```python
from build123d import *

# Parameters (mm, degrees)
BASPROSKE_W          = 4
BASPROSKE_H          = 12.375
TOOTHCUT_DEPTH       = 18.952193459
TEETHCUTS_COUNT      = 20
M2_CLEARANCE_HOLE1_D = 2.2
SKETCH3_R            = 2.5
CUT_EXTRUDE1_DEPTH   = 1


with BuildPart() as part:
    # BasProSke → Base-Revolve (revolve)
    with BuildSketch(Plane(origin=(0, 0, 0), x_dir=(1, 0, 0), z_dir=(0, 1, 0)), mode=Mode.PRIVATE) as base_revolve_sk:
        with Locations((2, 6.1875)):
            Rectangle(BASPROSKE_W, BASPROSKE_H)
    revolve(base_revolve_sk.sketch.rotate(Axis((-10, 0, 0), (1, 0, 0)), 180), axis=Axis((-10, 0, 0), (1, 0, 0)))

    # TooCutSke → ToothCut (cut, through all)
    with BuildSketch(Plane(origin=(0, 0, 0), x_dir=(0, 0, -1), z_dir=(1, 0, 0))):
        with BuildLine():
            ThreePointArc((0.561279811, 9.826733564), (0, 9.84275), (-0.561279811, 9.826733564))
            ThreePointArc((-0.561279811, 9.826733564), (-0.925277854, 11.14210546), (-1.666860651, 12.287859689))
            ThreePointArc((-1.666860651, 12.287859689), (0, 12.4004), (1.666860651, 12.287859689))
            ThreePointArc((1.666860651, 12.287859689), (0.925277854, 11.14210546), (0.561279811, 9.826733564))
        make_face()
    toothcut = extrude(amount=TOOTHCUT_DEPTH, mode=Mode.SUBTRACT)

    # TeethCuts: ToothCut ×20 about axis
    teethcuts_axis = Axis((0, 0, 0), (1, 0, 0))
    for i in range(1, TEETHCUTS_COUNT):
        add(toothcut.rotate(teethcuts_axis, i * 360 / TEETHCUTS_COUNT), mode=Mode.SUBTRACT)

    # M2 Clearance Hole1 (through all)
    with Locations(Plane(origin=(4, 0, 0), x_dir=(0, 0, -1), z_dir=(1, 0, 0))):
        with Locations((0, 0)):
            Hole(M2_CLEARANCE_HOLE1_D / 2)

    # Sketch3 → Cut-Extrude1 (cut)
    with BuildSketch(Plane(origin=(4, 0, 0), x_dir=(0, 0, -1), z_dir=(1, 0, 0))):
        Circle(SKETCH3_R)
    extrude(amount=-CUT_EXTRUDE1_DEPTH, mode=Mode.SUBTRACT)


solid = part.part
```
Model file for the job. Use its own axes, mm. A direction names the side the tool comes from. Round coordinates to 2 decimals unless told otherwise and drop trailing zeros. Write each loop counter-clockwise with the first axis right and the second up, starting at its lowest first coordinate (ties: lowest second). Pieces come first, ordered by that corner, then holes. Notation, with made-up numbers: (88, -28.5) - (107, -28.5) arc R34 ccw to (107, 7.5) - close; hole circle Ø2 at (61.25, 79). An arc over 180 degrees is marked (long way). Use CSV: the item, a comma, the result in double quotes. Start each with the question number.
Item 1: Band-saw the part on D-D (z = -4.5). Write the cut outline in (x, y).
Item 2: Band-saw the part on C-C (y = -4.25). Write the cut outline in (x, z).
Item 3: Band-saw the part on A-A (y = 0). Write the cut outline in (x, z), and give its area (3 significant figures).
Item 4: Drill centre lines: L1, parallel to Z at x = 1, y = 10.25; L2, parallel to Z at x = 1.6, y = 8.5; L3, parallel to Y at x = 1.45, z = 9.75. Where is each one in solid material? Low to high. Write a range as [from, to].
Item 5: Two-plate mould, pull along Z, no slides. Class faces 1 (the face through (1.972, 4.326, 10.314)), 2 (the face through (1.972, 2.563, -10.886)): released by +Z, released by -Z, zero draft, split by the parting line, or undercut.
Item 6: Pin check, flat tips, straight feed: P1, Ø3, axis at y = -5.5, z = 0, coming from the -X side; P2, Ø1, axis at x = 1.5, z = 7, coming from the -Y side; P3, Ø1.8, axis at y = 0, z = 0, coming from the -X side. Stop position of each tip, or through.
Item 7: Tool access for faces 3 (the face through (1.97, -11.11, -0.91)), 4 (the face through (1.972, -7.968, -5.779)), 5 (the face through (1.97, 11.11, 0.91)): list every direction of +Z, -Z, +X, -X, +Y, -Y with a clear straight run to the whole face (end or side of a thin tool).
Checked values:
1,outline,"(0, -10.5) - (4, -10.5) - (4, 10.5) - (0, 10.5) - close"
2,outline,"(0, -10.23) - (4, -10.23) - (4, 10.23) - (0, 10.23) - close"
3,outline,"(0, -9.84) - (4, -9.84) - (4, -2.5) - (3, -2.5) - (3, -1.1) - (0, -1.1) - close; (0, 1.1) - (3, 1.1) - (3, 2.5) - (4, 2.5) - (4, 9.84) - (0, 9.84) - close"
3,area,"67.1 mm²"
4,L1,"z = [-5.89, -4.27], [-2.59, -0.63], [0.63, 2.59], [4.27, 5.89]"
4,L2,"z = [-8.95, -7.35], [-5.44, 5.44], [7.35, 8.95]"
4,L3,"y = [-5.84, -3.89], [-2.54, 2.54], [3.89, 5.84]"
5,face 1,"released by +Z"
5,face 2,"undercut"
6,P1,"stops at x = 0"
6,P2,"stops at y = -8.58"
6,P3,"passes through"
7,face 3,"+X, -X, -Y"
7,face 4,"+X, -X"
7,face 5,"+X, -X, +Y"
